Input: part model. Units: mm. Frame: model coordinates. A direction names the side the tool comes from. Give positions to 0.01 mm unless a question says otherwise; leave off trailing zeros. Loops run counter-clockwise (first coordinate to the right, second up) from the corner with the lowest first, then second, coordinate; pieces in that order, holes last. Notation, with made-up numbers: M -27,-4.5 L -11,-4.5 A31 ccw -11,22.5 Z; hole C -36.5,77.5 d7. An arc over 180 degrees is marked long. One line per item, written item: value. Start each with the question number.
(1) Section C-C on y = -2.5. Output: boundary loops of the cut face in (x, z).
(2) Access query for faces 5 (the cylindrical face through (12.48, -31.54, -15.17)), 6 (the cylindrical face through (2.03, -36.44, -19.69)), 7 (the flat face through (0.6, -40.867, 0.4)). Directions: +Z, -Z, +X, -X, +Y, -Y. A direction counts if a zero-diameter tool reaches every point of the face in a straight line with its end or side. Return the directions, or none.
(3) Section B-B on x = 18.5. Output: boundary loops of the cut face in (y, z) (3 decimals).
(4) Ray query, line 1 along Y through (x, z) = (11.25, -13); line 2 along X through (y, z) = (-34.5, 5); line 3 along X through (y, z) = (-41, 13). Return the intervals inside material, ascending. Write a range as from..to.
(5) Pin query (flat end, axial travel): P1, Ø3, axis at x = 1.5, z = -7.5, coming from the -Y side; P2, Ø2, axis at x = 13.5, y = -29.5, coming from the -Z side; P3, Ø4.5, axis at y = -17.47, z = -19.95, coming from the +X side; P4, Ø2.5, axis at y = -44, z = 5.5, coming from the -X side. Return the tip coordinate at first contact, or that it passes through.
(6) Section A-A on y = -31.5. Output: boundary loops of the cut face in (x, z).
(7) Pull-direction query (Z, two-part tool) for faces 1 (the flat face through (2, -22, 31)), 2 (the cylindrical face through (2.03, -24.42, -17.86)), 3 (the flat face through (3, -43, -17.5)), 4 (the flat face through (2.3, -45, 0)); classes: released by +Z, released by -Z, zero draft, split by the parting line, or undercut.
Autodesk Inventor part; units mm, degrees
ref_plane "YZ Plane" through (0, 0, 0) normal (1, 0, 0) x (0, 1, 0)
ref_plane "XZ Plane" through (0, 0, 0) normal (0, 1, 0) x (-1, 0, 0)
ref_plane "XY Plane" through (0, 0, 0) normal (0, 0, 1) x (1, 0, 0)
sketch "Sketch1" plane through (0, 0, 0) normal (1, 0, 0) x (0, 1, 0)
  spline S0 degree 3 poles (-5.8666, 35) (13.8832, 21.2522) (-10.0462, -16.0043) (8.551, -35) knots 1 1 1 1 2 2 2 2
  line L0 (-5.8666, 35) -> (13.8832, 21.2522) construction
  line L1 (13.8832, 21.2522) -> (-10.0462, -16.0043) construction
  line L2 (-10.0462, -16.0043) -> (8.551, -35) construction
  line L3 (0, 65.172) -> (0, -65.172) construction
  line L4 (43.74, 0) -> (-43.74, 0) construction
  line L5 (-5.8666, 35) -> (-40.8666, 35)
  line L6 (-40.8666, 35) -> (-40.8666, 31)
  line L7 (-40.8666, 31) -> (-1.7165, 31)
  line L8 (-40.8666, 31) -> (-40.8666, -35)
  line L9 (-40.8666, -35) -> (8.551, -35)
  line L10 (-40.8666, -31) -> (5.392, -31)
  point P0 (0, 0)
  point P1 (0, 0)
  point P2 (-1.7165, 31)
  point P3 (0, 0)
  point P4 (0, 0)
  point P5 (0, 0)
  dimension "d0" = 35
  dimension "d1" = 4
  dimension "d2" = 4
extrude "Extrusion1" add sketch "Sketch1" along normal blind 4 contours S0 L10 L8 L7
sketch "Sketch3" plane through (0, -40.8666, -31) normal (0, -1, 0) x (1, 0, 0)
  line L0 (2.3, 48.5) -> (4, 48.5)
  line L1 (4, 48.5) -> (4, 13.5)
  line L2 (4, 13.5) -> (2.3, 13.5)
  line L3 (2.3, 13.5) -> (2.3, 48.5)
  line L4 (0, 62) -> (0, 0)
  line L5 (0, 0) -> (4, 0)
  line L6 (4, 62) -> (4, 0)
  line L7 (0, 62) -> (4, 62)
  point P0 (0, 31)
  point P1 (4, 31)
  dimension "d5" = 1.7
  dimension "d6" = 35
extrude "Extrusion2" add sketch "Sketch3" along normal blind 4.9 contours L0 L1 L2 L3
sketch "Sketch4" plane through (4, 0, 0) normal (1, 0, 0) x (0, 0, -1)
  circle A0 centre (12.8601, -10.8083) radius 2.425
  circle A1 centre (12.8601, -30.8083) radius 2.425
  line L0 (12.8601, -10.8083) -> (12.8601, -30.8083) construction
  circle A2 centre (-17.6399, -20.8083) radius 2.3037
  point P0 (0, 0)
  dimension "d11" = 4.85
  dimension "d12" = 4.85
  dimension "d13" = 20
  dimension "d14" = 4.6075
  dimension "d15" = 30.5
extrude "Extrusion3" add sketch "Sketch4" along normal blind 17.2
chamfer "Chamfer1" distance 1.5 angle 45 1 edges at (2.3, -40.8666, 0)
sketch "Sketch5" plane through (4, 0, 0) normal (1, 0, 0) x (0, 0, -1)
  arc A0 (17.8302, -18.7899) -> (16.2318, -18.8201) centre (17.0282, -18.6552) ccw construction
  arc A1 (18.4232, -18.8896) -> (15.643, -18.942) centre (17.0282, -18.6552) ccw
  arc A2 (17.2372, -18.6903) -> (16.8207, -18.6981) centre (17.0282, -18.6552) ccw
  arc A3 (17.2372, -18.6903) -> (18.4232, -18.8896) centre (17.8302, -18.7899) ccw
  arc A4 (15.643, -18.942) -> (16.8207, -18.6981) centre (16.2318, -18.8201) ccw
  arc A5 (17.1142, -21.1556) -> (16.3411, -22.5549) centre (16.5965, -21.7828) ccw construction
  arc A6 (17.497, -20.6919) -> (16.1523, -23.1258) centre (16.5965, -21.7828) ccw
  arc A7 (16.7314, -21.6193) -> (16.5299, -21.984) centre (16.5965, -21.7828) ccw
  arc A8 (16.7314, -21.6193) -> (17.497, -20.6919) centre (17.1142, -21.1556) ccw
  arc A9 (16.1523, -23.1258) -> (16.5299, -21.984) centre (16.3411, -22.5549) ccw
  arc A10 (18.8049, -22.9585) -> (19.6302, -24.3277) centre (19.0892, -23.7205) ccw construction
  arc A11 (18.5947, -22.3952) -> (20.0302, -24.7766) centre (19.0892, -23.7205) ccw
  arc A12 (19.0151, -23.5219) -> (19.2302, -23.8787) centre (19.0892, -23.7205) ccw
  arc A13 (19.0151, -23.5219) -> (18.5947, -22.3952) centre (18.8049, -22.9585) ccw
  arc A14 (20.0302, -24.7766) -> (19.2302, -23.8787) centre (19.6302, -24.3277) ccw
  arc A15 (21.2117, -22.3958) -> (22.81, -22.3656) centre (22.0137, -22.5305) ccw construction
  arc A16 (20.6187, -22.2961) -> (23.3988, -22.2437) centre (22.0137, -22.5305) ccw
  arc A17 (21.8047, -22.4954) -> (22.2212, -22.4875) centre (22.0137, -22.5305) ccw
  arc A18 (21.8047, -22.4954) -> (20.6187, -22.2961) centre (21.2117, -22.3958) ccw
  arc A19 (23.3988, -22.2437) -> (22.2212, -22.4875) centre (22.81, -22.3656) ccw
  arc A20 (21.9277, -20.0301) -> (22.7007, -18.6308) centre (22.4454, -19.4029) ccw construction
  arc A21 (21.5449, -20.4938) -> (22.8895, -18.0599) centre (22.4454, -19.4029) ccw
  arc A22 (22.3105, -19.5663) -> (22.5119, -19.2017) centre (22.4454, -19.4029) ccw
  arc A23 (22.3105, -19.5663) -> (21.5449, -20.4938) centre (21.9277, -20.0301) ccw
  arc A24 (22.8895, -18.0599) -> (22.5119, -19.2017) centre (22.7007, -18.6308) ccw
  arc A25 (20.2369, -18.2272) -> (19.4116, -16.858) centre (19.9526, -17.4652) ccw construction
  arc A26 (20.4471, -18.7905) -> (19.0116, -16.4091) centre (19.9526, -17.4652) ccw
  arc A27 (20.0267, -17.6638) -> (19.8117, -17.307) centre (19.9526, -17.4652) ccw
  arc A28 (20.0267, -17.6638) -> (20.4471, -18.7905) centre (20.2369, -18.2272) ccw
  arc A29 (19.0116, -16.4091) -> (19.8117, -17.307) centre (19.4116, -16.858) ccw
  arc A30 (23.0405, -38.7872) -> (16.269, -38.8619) centre (19.6983, -42.7704) ccw construction
  arc A31 (23.7678, -37.9205) -> (15.5229, -38.0114) centre (19.6983, -42.7704) ccw
  arc A32 (22.3133, -39.6539) -> (17.0152, -39.7123) centre (19.6983, -42.7704) ccw
  arc A33 (22.3133, -39.6539) -> (23.7678, -37.9205) centre (23.0405, -38.7872) ccw
  arc A34 (15.5229, -38.0114) -> (17.0152, -39.7123) centre (16.269, -38.8619) ccw
  point P0 (0, 0)
  point P1 (19.5209, -20.5928)
  dimension "d30" = 360
extrude "Extrusion4" cut sketch "Sketch5" against normal blind 4
sketch "Sketch6" plane through (4, 0, 0) normal (1, 0, 0) x (0, 0, -1)
  line L0 (-17.5, -40.8666) -> (17.5, -40.8666)
  circle A0 centre (0, -43.1166) radius 1.575
  line L1 (17.5, -40.8666) -> (17.5, -45.7666)
  point P0 (0, 0)
  dimension "d32" = 3.15
  dimension "d33" = 2.25
  dimension "d36" = 17.5
extrude "Extrusion5" cut sketch "Sketch6" against normal blind 4
equation "\"d11\" = d12"
equation "\"d14\" = 0.95 * d12"
properties part number "Case Right"
Output values:
1. outline: M 0,-31 L 4,-31 L 4,31 L 0,31 Z
2. face 5: +X
2. face 6: +X, -X
2. face 7: -X, -Y
3. outline: C -30.808,-12.86 d4.85; C -20.808,17.64 d4.607; C -10.808,-12.86 d4.85
4. line 1: y = -33.23..-28.39, -13.23..-8.39
4. line 2: x = 0..4
4. line 3: x = 0.93..4
5. P1: stops at y = -45.77
5. P2: stops at z = -15.27
5. P3: stops at x = 4
5. P4: stops at x = 2.3
6. outline: M 0,-31 L 4,-31 L 4,-15.18 L 21.2,-15.18 L 21.2,-10.54 L 4,-10.54 L 4,31 L 0,31 Z
7. face 1: released by +Z
7. face 2: undercut
7. face 3: released by -Z
7. face 4: zero draft
